Check sheet for the modelled part. Datum: model origin and axes. Units: mm. Round coordinates to 2 decimals unless told otherwise and drop trailing zeros. Order: outer loops, then holes, each group sorted by start corner. A loop starts at its lowest first (then second) coordinate and runs counter-clockwise, first axis right, second up. Notation, with made-up numbers: (69.25, 54.25) -> (81.25, 54.25) arc R11 ccw to (81.25, 59.25) -> close; hole circle Ø11 at (11.5, 40.5). An arc over 180 degrees is marked (long way). Answer in a Markdown table with one row per item.
from build123d import *

# Parameters (mm, degrees)
BOSS_EXTRUDE1_DEPTH     = 256.54
CUT_EXTRUDE1_REACH      = 815.442
SKETCH2_R               = 11.1125
CUT_EXTRUDE2_DEPTH      = 814.446927228
CUT_EXTRUDE2_DEPTH_BACK = 814.446927228
FILLET1_R               = 12.7


with BuildPart() as part:
    # Sketch1 → Boss-Extrude1 (new body)
    with BuildSketch(Plane.XY):
        Polygon((-443.965929871, -405.988484906), (-553.446258124, -541.061617166), (-558.379343621, -537.063221553), (-448.899015368, -401.990089292), align=None)
    extrude(amount=BOSS_EXTRUDE1_DEPTH)

    # Sketch2 → Cut-Extrude1 (cut, up to next)
    with BuildSketch(Plane(origin=(-74.278193829, 60.204430788, 0), x_dir=(0, 0, 1), z_dir=(-0.7768638577795597, 0.6296686005160651, 0)), mode=Mode.PRIVATE) as cut_extrude1_sk1:
        with Locations(Location((213.995, -645.749186336, 0), (0, 0, 270))):
            Circle(SKETCH2_R)
    cut_extrude1_tool1 = extrude(cut_extrude1_sk1.sketch, amount=-CUT_EXTRUDE1_REACH, mode=Mode.PRIVATE) & part.part
    # Sketch2 → Cut-Extrude1 (cut, up to next)
    with BuildSketch(Plane(origin=(-74.278193829, 60.204430788, 0), x_dir=(0, 0, 1), z_dir=(-0.7768638577795597, 0.6296686005160651, 0)), mode=Mode.PRIVATE) as cut_extrude1_sk2:
        with Locations(Location((36.195, -645.749186336, 0), (0, 0, 270))):
            Circle(SKETCH2_R)
    cut_extrude1_tool2 = extrude(cut_extrude1_sk2.sketch, amount=-CUT_EXTRUDE1_REACH, mode=Mode.PRIVATE) & part.part
    add(cut_extrude1_tool1.solids().sort_by_distance((-480.88618, -441.454773, 213.995))[0], mode=Mode.SUBTRACT)
    add(cut_extrude1_tool2.solids().sort_by_distance((-480.88618, -441.454773, 36.195))[0], mode=Mode.SUBTRACT)

    # Sketch3 → Cut-Extrude2 (cut, two sides: drawn at the far end of the back side and taken through both)
    with BuildSketch(Plane(origin=(-69.345108332, 56.206035175, 0), x_dir=(0, 0, -1), z_dir=(0.7768638577795598, -0.6296686005160651, 0)).offset(-CUT_EXTRUDE2_DEPTH_BACK)):
        Polygon((269.008566256, -1124.880370714), (-205.74, -768.818946022), (-256.54, -730.718946022), (-731.288566256, -374.65752133), (-1443.411415639, -1324.154653842), (-443.114283128, -2074.377503225), align=None)
    extrude(amount=CUT_EXTRUDE2_DEPTH + CUT_EXTRUDE2_DEPTH_BACK, mode=Mode.SUBTRACT)

    # Fillet1
    fillet1_edges = [part.edges().sort_by_distance(p)[0] for p in [
        (-531.922427193, -509.463906378, 256.54),
        (-446.432472619, -403.989287099, 256.54),
        (-555.912800873, -539.062419359, 205.74),
        (-446.432472619, -403.989287099, 0),
    ]]
    fillet(fillet1_edges, radius=FILLET1_R)


solid = part.part
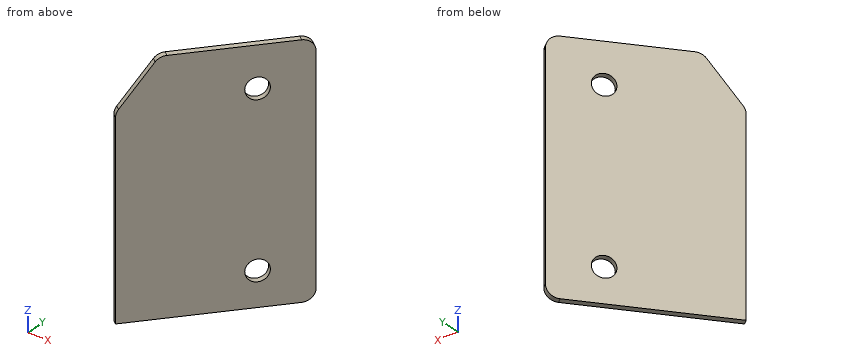
Item 1: Cross-section at A-A (z = 29). Record the boundary of the cut face in (x, y).
Result sheet:
| item | result |
|---|---|
| outline | (-558.38, -537.06) -> (-553.45, -541.06) -> (-481.29, -452.03) -> (-486.22, -448.03) -> close; (-475.55, -434.88) -> (-470.62, -438.87) -> (-443.97, -405.99) -> (-448.9, -401.99) -> close |
Item 2: Cross-section at D-D (z = 147.5). Record the boundary of the cut face in (x, y), and give its area (3 significant figures).
Result sheet:
| item | result |
|---|---|
| outline | (-558.38, -537.06) -> (-553.45, -541.06) -> (-443.97, -405.99) -> (-448.9, -401.99) -> close |
| area | 1,100 mm^2 |
Item 3: Depth check by flat-ended pin: P1, Ø5, axis at x = -505.5, z = 82.5, coming from the +Y side; P2, Ø12, axis at y = -467, z = 91, coming from the -X side; P3, Ø8, axis at x = -532, z = 169, coming from the +Y side. Enter the tip coordinate at first touch or a pass-through.
Result sheet:
| item | result |
|---|---|
| P1 | stops at y = -468.74 |
| P2 | stops at x = -506.45 |
| P3 | stops at y = -499.58 |
Item 4: Cross-section at B-B (y = -444.5). State how many separate pieces and enclosed holes the cut face has, and give its area (3 significant figures).
Result sheet:
| item | result |
|---|---|
| separate pieces | 3 |
| enclosed holes | 0 |
| area | 1,740 mm^2 |
Item 5: Scan lines: line 1 (X direction, y = -438, z = 131); line 2 (X direction, y = -524.5, z = 151.5); line 3 (Z direction, x = -543, y = -520.5). Record each from-to range of solid material in increasing order. Write a range as [from, to].
Result sheet:
| item | result |
|---|---|
| line 1 | x = [-478.09, -469.91] |
| line 2 | x = [-548.2, -540.02] |
| line 3 | z = [0, 235.81] |
